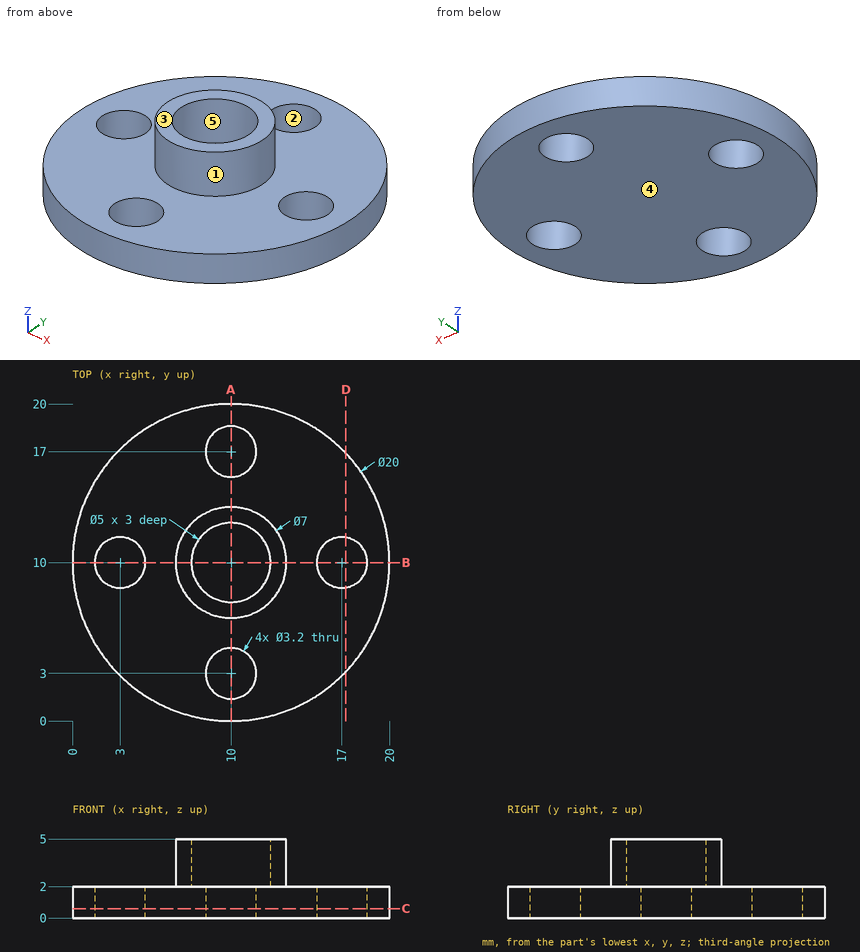
Verification items for this drawing (mm, ordinates from the low corner). A direction names the side the tool comes from. Give positions to 0.01 mm unless a question says otherwise; leave off trailing zeros. Order: outer loops, then holes, each group sorted by start corner. A loop starts at its lowest first (then second) coordinate and runs counter-clockwise, first axis right, second up. Notation, with made-up numbers: M 87.5,39 L 134.5,39 A10 cw 134.5,45 Z; hole C -4,39.25 d5. An arc over 180 degrees is marked long. Use a Markdown table: item, result.
Item 1: Section check A-A (x = 10). Record the cut outline in (y, z), and give its area (3 significant figures).
Answers follow:
| item | result |
|---|---|
| outline | M 0,0 L 1.4,0 L 1.4,2 L 0,2 Z; M 4.6,0 L 15.4,0 L 15.4,2 L 13.5,2 L 13.5,5 L 12.5,5 L 12.5,2 L 7.5,2 L 7.5,5 L 6.5,5 L 6.5,2 L 4.6,2 Z; M 18.6,0 L 20,0 L 20,2 L 18.6,2 Z |
| area | 33.2 mm2 |
Item 2: Material ranges on line 1 along Z through (x, y) = (13.25, 18.25); line 2 along X through (y, z) = (16.75, 1.8); line 3 along Y through (x, z) = (12, 3.8), recorded low to high.
Answers follow:
| item | result |
|---|---|
| line 1 | z = 0 to 2 |
| line 2 | x = 2.62 to 8.42, 11.58 to 17.38 |
| line 3 | y = 7.13 to 8.5, 11.5 to 12.87 |
Item 3: Section check D-D (x = 17.25). Record the cut outline in (y, z).
Answers follow:
| item | result |
|---|---|
| outline | M 3.11,0 L 8.42,0 L 8.42,2 L 3.11,2 Z; M 11.58,0 L 16.89,0 L 16.89,2 L 11.58,2 Z |
Item 4: Draft check along Y on the marked faces 1, 2 and 3. Enter one of: +Y half, -Y half, draft (parallel to the pull), parting line (faces both ways), or undercut.
Answers follow:
| item | result |
|---|---|
| face 1 | parting line |
| face 2 | undercut |
| face 3 | draft |
Item 5: Depth check by flat-ended pin: P1, Ø4, axis at x = 17, y = 8.5, coming from the +Z side; P2, Ø2.5, axis at x = 10, y = 17, coming from the -Z side; P3, Ø1.5, axis at y = 8.5, z = 1, coming from the -X side. Enter the tip coordinate at first touch or a pass-through.
Answers follow:
| item | result |
|---|---|
| P1 | stops at z = 2 |
| P2 | passes through |
| P3 | stops at x = 0.03 |
Item 6: Tool access check on the marked faces 4 and 5. Record the directions out of +Z, -Z, +X, -X, +Y, -Y that give a thin tool (end or side, any length) a straight path to the whole face; none if there is none.
Answers follow:
| item | result |
|---|---|
| face 4 | -Z, +X, -X, +Y, -Y |
| face 5 | +Z |
Item 7: Section check C-C (z = 0.6). Record the cut outline in (x, y).
Answers follow:
| item | result |
|---|---|
| outline | C 10,10 d20; hole C 3,10 d3.2; hole C 10,3 d3.2; hole C 10,17 d3.2; hole C 17,10 d3.2 |
